Input: dimensioned drawing with shaded views. Units: mm. Origin: part minimum x, y, z. A direction names the side the tool comes from. Give positions to 0.01 mm unless a question says otherwise; leave off trailing zeros. Loops run counter-clockwise (first coordinate to the right, second up) from the corner with the lowest first, then second, coordinate; pieces in that order, holes last. Notation, with made-up numbers: M -39.5,-39.75 L 19.5,-39.75 A9 ccw 19.5,-23.75 Z; hole C 23,51 d9. An arc over 180 degrees is marked long. Answer in a Markdown table with one row per item.
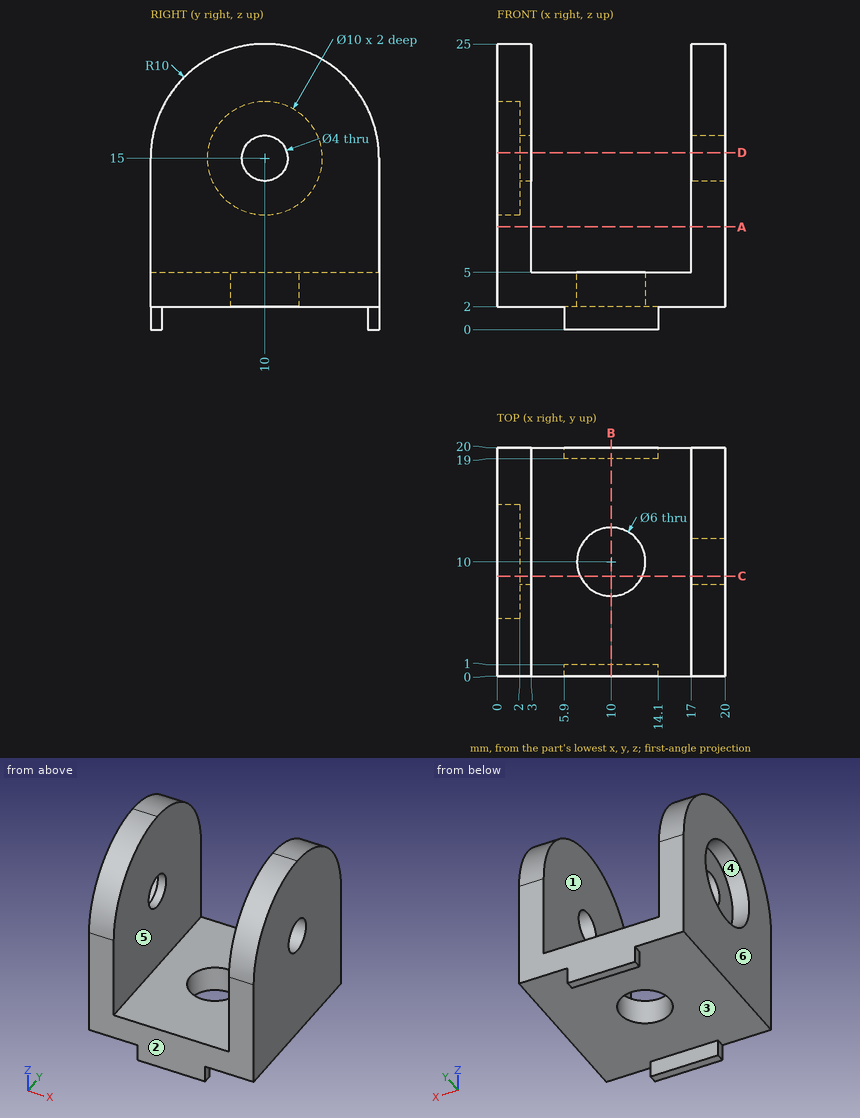
Q1. Section query B-B (x = 10). Output: boundary loops of the cut face in (y, z).
Values follow:
| item | result |
|---|---|
| outline | M 0,0 L 1,0 L 1,2 L 7,2 L 7,5 L 0,5 Z; M 13,2 L 19,2 L 19,0 L 20,0 L 20,5 L 13,5 Z |
Q2. Section query D-D (z = 15.5). Output: boundary loops of the cut face in (x, y), plus the area to 3 significant figures.
Values follow:
| item | result |
|---|---|
| outline | M 0,0.01 L 3,0.01 L 3,8.06 L 2,8.06 L 2,5.03 L 0,5.03 Z; M 0,14.97 L 2,14.97 L 2,11.94 L 3,11.94 L 3,19.99 L 0,19.99 Z; M 17,0.01 L 20,0.01 L 20,8.06 L 17,8.06 Z; M 17,11.94 L 20,11.94 L 20,19.99 L 17,19.99 Z |
| area | 84.5 mm^2 |
Q3. Ray query, probe 1 along X at (y, z) = (5, 8); probe 2 along X at (y, z) = (10.75, 10.5); probe 3 along Y at (x, z) = (18.3, 15). Return the intervals inside material, ascending. Write a range as from..to.
Values follow:
| item | result |
|---|---|
| probe 1 | 0..3, 17..20 |
| probe 2 | 2..3, 17..20 |
| probe 3 | 0..8, 12..20 |
Q4. Section query C-C (y = 8.75). Output: boundary loops of the cut face in (x, z).
Values follow:
| item | result |
|---|---|
| outline | M 0,2 L 7.27,2 L 7.27,5 L 3,5 L 3,13.44 L 2,13.44 L 2,10.16 L 0,10.16 Z; M 0,19.84 L 2,19.84 L 2,16.56 L 3,16.56 L 3,24.92 L 0,24.92 Z; M 12.73,2 L 20,2 L 20,13.44 L 17,13.44 L 17,5 L 12.73,5 Z; M 17,16.56 L 20,16.56 L 20,24.92 L 17,24.92 Z |
Q5. Section query A-A (z = 9). Output: boundary loops of the cut face in (x, y), plus the area to 3 significant figures.
Values follow:
| item | result |
|---|---|
| outline | M 0,0 L 3,0 L 3,20 L 0,20 Z; M 17,0 L 20,0 L 20,20 L 17,20 Z |
| area | 120 mm^2 |
Q6. Mould query, pull axis Y, two halves, no side actions, for the marked faces 1, 2 and 3. Classes: +Y half, -Y half, draft (parallel to the pull), parting line (faces both ways), or undercut.
Values follow:
| item | result |
|---|---|
| face 1 | draft |
| face 2 | -Y half |
| face 3 | undercut |
Q7. Contact query for flat-ended pins moving along their axis: pin 1 Ø4 at (x, z) = (6, 11) entering from -Y; pin 2 Ø6 at (x, y) = (10, 5) entering from +Z; pin 3 Ø0.5 at (y, z) = (0.5, 0.5) entering from +X; pin 4 Ø1.1 at (y, z) = (19.5, 1) entering from -X. Output: stop coordinate, or through.
Values follow:
| item | result |
|---|---|
| pin 1 | through |
| pin 2 | z = 5 |
| pin 3 | x = 14.1 |
| pin 4 | x = 5.9 |
Q8. Reachability of the marked faces 4, 5 and 6 from +Z, -Z, +X, -X, +Y, -Y: full face, straight path, thin tool, end or side. Return the list, or none.
Values follow:
| item | result |
|---|---|
| face 4 | -X |
| face 5 | +Z, +Y, -Y |
| face 6 | +Z, -Z, -X, +Y, -Y |
